Geometry: final body of the model. Coordinates: model frame, mm. Give positions to 0.01 mm unless a question says otherwise; leave off trailing zeros. Write each loop counter-clockwise with the first axis right and the second up, starting at its lowest first coordinate (ties: lowest second). Pieces come first, ordered by that corner, then holes. Notation, with made-up numbers: M 25.25,21.25 L 51.25,21.25 A23 ccw 51.25,37.25 Z; hole C -26,-18 d5. An arc over 180 degrees is marked long. Use a Markdown table: item, result. Add a question column.
1) Draft query along X for faces 1 (the flat face through (125, -2, 5)), 2 (the cylindrical face through (7.493, 0.33, 4.93)), 3 (the cylindrical face through (-42.253, 0.121, 4.93)), 4 (the flat face through (-2, -125, 5)). Return one class per face: +X half, -X half, draft (parallel to the pull), parting line (faces both ways), or undercut.
2) Section A-A on x = 0. Return the cut outline in (y, z), then the cut area to 3 significant figures.
3) Line query: line 1 (Y direction, x = 45, z = 2); line 2 (Y direction, x = 0, z = 3); line 3 (X direction, y = 3.5, z = 8.5). Output: solid intervals per line, ascending.
```python
from build123d import *

# Parameters (mm, degrees)
SKIZZE1_W                        = 250
SKIZZE1_H                        = 250
AUFSATZ_LINEAR_AUSTRAGEN1_DEPTH  = 10
F_5_5_5_5_DURCHMESSER_BOHRUNG1_D = 5.5
F_15_0_15_DURCHMESSER_BOHRUNG1_D = 15


with BuildPart() as part:
    # Skizze1 → Aufsatz-Linear austragen1 (new body)
    with BuildSketch(Plane.XY):
        Rectangle(SKIZZE1_W, SKIZZE1_H)
    extrude(amount=AUFSATZ_LINEAR_AUSTRAGEN1_DEPTH)

    # Ø5.5 (5.5) Durchmesser Bohrung1 (through all)
    with Locations(Plane.XY.offset(10)):
        with Locations((45, 0), (-45, 0)):
            Hole(F_5_5_5_5_DURCHMESSER_BOHRUNG1_D / 2)

    # Ø15.0 (15) Durchmesser Bohrung1 (through all)
    with Locations(Plane.XY.offset(10)):
        with Locations((0, 0)):
            Hole(F_15_0_15_DURCHMESSER_BOHRUNG1_D / 2)


solid = part.part
```
Found:
| question | item | result |
|---|---|---|
| 1 | face 1 | +X half |
| 1 | face 2 | undercut |
| 1 | face 3 | undercut |
| 1 | face 4 | draft |
| 2 | outline | M -125,0 L -7.5,0 L -7.5,10 L -125,10 Z; M 7.5,0 L 125,0 L 125,10 L 7.5,10 Z |
| 2 | area | 2,350 mm² |
| 3 | line 1 | -125 to -2.75, 2.75 to 125 |
| 3 | line 2 | -125 to -7.5, 7.5 to 125 |
| 3 | line 3 | -125 to -6.63, 6.63 to 125 |
